CAD build for the part. Positions are in the model's coordinates, mm. A direction names the side the tool comes from. Coordinates: 2 decimals unless noted, no trailing zeros. Loops run counter-clockwise (first coordinate to the right, second up) from the corner with the lowest first, then second, coordinate; pieces in that order, holes last.
1) Saw through at B-B, the plane x = 0. Write the cut outline in (y, z), and give its area (3 significant figures).
2) Saw through at C-C, the plane y = 3.5. Give the number of separate pieces and of enclosed holes in the cut face, and give its area (3 significant figures).
3) Wall check: line 1 along X through (y, z) = (4.2, 5); line 2 along Z through (x, y) = (0, 5.6); line 3 along X through (y, z) = (5.95, 0). Give the ranges that are in metal, low to high.
4) Which spindle directions (+Z, -Z, +X, -X, +Y, -Y) get a long thin tool onto all of the face, cutting with end or side? Do faces 1 (the flat face through (-5.3, 1, 5.5)), 2 (the flat face through (5.2, 1, 5.5)), 3 (the cylindrical face through (5, 6, 0)), 4 (the flat face through (-3.5, 3.7, 3.2)), 5 (the cylindrical face through (-4.672, 7.998, -0.176)). Say none if no direction does.
5) Pin check, flat tips, straight feed: pin 1 Ø0.8 at (x, y) = (-5, 0.5) entering from +Z; pin 2 Ø0.8 at (x, y) = (-5, 0.5) entering from -Z; pin 3 Ø1 at (x, y) = (-0.5, 3.5) entering from -Z. Stop position of each tip, or through.
6) Two-plate mould, pull along X, no slides. Class faces 6 (the flat face through (0, 3, 3.5)), 7 (the flat face through (0, 0, -7)), 8 (the conical face through (4.897, 8.154, -0.179)): +X half, -X half, draft (parallel to the pull), parting line (faces both ways), or undercut.
7) Saw through at A-A, the plane x = -1.5. Write the cut outline in (y, z), and give its area (3 significant figures).
```python
from build123d import *

# Parameters (mm, degrees)
PADSKE_R             = 6
PAD_DEPTH            = 6
HOLE_DEPTH           = 18.334935823
HOLE_DEPTH_BACK      = 18.334935823
HOLESKE_R            = 4
SCREWHOLE_DEPTH      = 18.334935823
SCREWHOLE_DEPTH_BACK = 18.334935823
SCREWHOLESKE_R       = 0.35
BOXSKE_W             = 7
BOXSKE_H             = 8
BOX_DEPTH            = 3.5
CUTSKE_W             = 26
CUTSKE_H             = 26
CUT_DEPTH            = 20
SCREWHOLE2SKE_R      = 0.35
SCREWHOLE2_DEPTH     = 18.334935823
SLOTSKE_W            = 1.5
SLOTSKE_H            = 1
SLOT_DEPTH           = 1
FLANGESLOTSKE_R      = 4.65
FLANGESLOT_DEPTH     = 0.7
EDGE_2_ANGLE         = 180
CHAMFER_2_SIZE       = 1
CHAMFER_2_SIZE2      = 4
CHAMFER2_SIZE        = 4
CHAMFER2_SIZE2       = 1


with BuildPart() as part:
    # BodySke → Body (revolve)
    with BuildSketch(Plane(origin=(0, 0, 0), x_dir=(1, 0, 0), z_dir=(0, 1, 0)), mode=Mode.PRIVATE) as body_sk:
        Polygon((4.5, 0), (4.5, 11.5), (4.3, 11.5), (2.298163712, 6), (-2.298163712, 6), (-4.3, 11.5), (-4.5, 11.5), (-4.5, 0), align=None)
    revolve(body_sk.sketch.rotate(Axis((-4.5, 0, 0), (1, 0, 0)), 180), axis=Axis((-4.5, 0, 0), (1, 0, 0)))

    # BoldSke → Bold (revolve)
    with BuildSketch(Plane(origin=(0, 0, 0), x_dir=(1, 0, 0), z_dir=(0, 1, 0)), mode=Mode.PRIVATE) as bold_sk:
        Polygon((-2.298163712, 6), (2.298163712, 6), (2.844119063, 7.5), (-2.844119063, 7.5), align=None)
    revolve(bold_sk.sketch.rotate(Axis((0, 0, 0), (1, 0, 0)), 180), axis=Axis((0, 0, 0), (1, 0, 0)))

    # PadSke → Pad (add, symmetric)
    with BuildSketch(Plane(origin=(0, 0, 0), x_dir=(0, 0, -1), z_dir=(1, 0, 0))):
        Circle(PADSKE_R)
    extrude(amount=PAD_DEPTH, both=True)

    # HoleSke → Hole (cut, two sides: drawn at the far end of the back side and taken through both)
    with BuildSketch(Plane(origin=(0, 0, 0), x_dir=(0, 0, -1), z_dir=(1, 0, 0)).offset(-HOLE_DEPTH_BACK)):
        Circle(HOLESKE_R)
    extrude(amount=HOLE_DEPTH + HOLE_DEPTH_BACK, mode=Mode.SUBTRACT)

    # ScrewHoleSke → ScrewHole (cut, two sides: drawn at the far end of the back side and taken through both)
    with BuildSketch(Plane(origin=(0, 0, 0), x_dir=(1, 0, 0), z_dir=(0, 1, 0)).offset(-SCREWHOLE_DEPTH_BACK)):
        with Locations(Location((0, 0, 0), (0, 0, 270))):
            Circle(SCREWHOLESKE_R)
    extrude(amount=SCREWHOLE_DEPTH + SCREWHOLE_DEPTH_BACK, mode=Mode.SUBTRACT)

    # BoxSke → Box (cut, symmetric)
    with BuildSketch(Plane.XY):
        Rectangle(BOXSKE_W, BOXSKE_H)
    extrude(amount=BOX_DEPTH, both=True, mode=Mode.SUBTRACT)

    # CutSke → Cut (cut)
    with BuildSketch(Plane(origin=(0, 0, 0), x_dir=(1, 0, 0), z_dir=(0, 1, 0))):
        Rectangle(CUTSKE_W, CUTSKE_H)
    extrude(amount=-CUT_DEPTH, mode=Mode.SUBTRACT)

    # ScrewHole2Ske → ScrewHole2 (cut, through all)
    with BuildSketch(Plane.XZ):
        with Locations(Location((0, -5, 0), (0, 0, 270))):
            Circle(SCREWHOLE2SKE_R)
        with Locations(Location((0, 5, 0), (0, 0, 270))):
            Circle(SCREWHOLE2SKE_R)
    extrude(amount=-SCREWHOLE2_DEPTH, mode=Mode.SUBTRACT)

    # SlotSke → Slot (cut)
    with BuildSketch(Plane.XZ):
        with Locations((-5.25, 5.5)):
            Rectangle(SLOTSKE_W, SLOTSKE_H)
        with Locations((5.25, 5.5)):
            Rectangle(SLOTSKE_W, SLOTSKE_H)
        with Locations((5.25, -5.5)):
            Rectangle(SLOTSKE_W, SLOTSKE_H)
        with Locations((-5.25, -5.5)):
            Rectangle(SLOTSKE_W, SLOTSKE_H)
    extrude(amount=-SLOT_DEPTH, mode=Mode.SUBTRACT)

    # FlangeSlotSke → FlangeSlot (cut)
    with BuildSketch(Plane(origin=(-3.5, 0, 0), x_dir=(0, 0, -1), z_dir=(1, 0, 0))):
        Circle(FLANGESLOTSKE_R)
    flangeslot = extrude(amount=-FLANGESLOT_DEPTH, mode=Mode.SUBTRACT)

    # FlangeSlot2: FlangeSlot across plane
    add(flangeslot.mirror(Plane(origin=(0, 0, 0), x_dir=(0, 0, 1), z_dir=(1, 0, 0))), mode=Mode.SUBTRACT)

    # EdgeSke → Edge 2 (revolve)
    with BuildSketch(Plane(origin=(0, 0, 0), x_dir=(1, 0, 0), z_dir=(0, 1, 0))):
        Polygon((4.5, 8), (4.840074414, 8), (5.75, 10.5), (5.75, 11.5), (4.5, 11.5), align=None)
        Polygon((-5.75, 11.5), (-4.5, 11.5), (-4.5, 8), (-4.840074414, 8), (-5.75, 10.5), align=None)
    revolve(axis=Axis((-4.5, 0, 0), (1, 0, 0)), revolution_arc=EDGE_2_ANGLE)

    # Chamfer 2
    chamfer_2_edges = [part.edges().sort_by_distance(p)[0] for p in [
        (4.3, 11.5, 0),
    ]]
    chamfer_2_side = [part.faces().sort_by_distance(p)[0] for p in [
        (4.4, 11.5, 0),
    ]]
    chamfer(chamfer_2_edges, length=CHAMFER_2_SIZE, length2=CHAMFER_2_SIZE2, reference=chamfer_2_side[0])

    # Chamfer2
    chamfer2_edges = [part.edges().sort_by_distance(p)[0] for p in [
        (-4.3, 11.5, 0),
    ]]
    chamfer2_side = [part.faces().sort_by_distance(p)[0] for p in [
        (-3.572059531, 9.5, 0),
    ]]
    chamfer(chamfer2_edges, length=CHAMFER2_SIZE, length2=CHAMFER2_SIZE2, reference=chamfer2_side[0])


solid = part.part
```
Data:
1. outline: (0, -7.5) arc R7.5 ccw to (5.26, -5.35) - (0, -5.35) - close; (0, -4.65) - (5.88, -4.65) arc R7.5 ccw to (7.49, -0.35) - (4, -0.35) - (4, -3.5) - (1.94, -3.5) arc R4 cw to (0, -4) - close; (0, 4) arc R4 cw to (1.94, 3.5) - (4, 3.5) - (4, 0.35) - (7.49, 0.35) arc R7.5 ccw to (5.88, 4.65) - (0, 4.65) - close; (0, 5.35) - (5.26, 5.35) arc R7.5 ccw to (0, 7.5) - close
1. area: 48.8 mm2
2. separate pieces: 2
2. enclosed holes: 2
2. area: 98.4 mm2
3. line 1: x = -4.5 to -0.35, 0.35 to 4.5
3. line 2: z = -4.65 to -0.35, 0.35 to 4.65
3. line 3: x = -6 to -0.35, 0.35 to 6
4. face 1: -X, -Y
4. face 2: +X, -Y
4. face 3: +X
4. face 4: -Y
4. face 5: -X
5. pin 1: stops at z = 11.5
5. pin 2: stops at z = -11.5
5. pin 3: stops at z = -6.87
6. face 6: undercut
6. face 7: draft
6. face 8: +X half
7. outline: (0, -7.5) arc R7.5 ccw to (0, 7.5) - (0, 4) arc R4 cw to (1.94, 3.5) - (4, 3.5) - (4, -3.5) - (1.94, -3.5) arc R4 cw to (0, -4) - close
7. area: 59.0 mm2
